Autodesk Inventor part; units mm, degrees
ref_plane "YZ Plane" through (0, 0, 0) normal (1, 0, 0) x (0, 1, 0)
ref_plane "XZ Plane" through (0, 0, 0) normal (0, 1, 0) x (-1, 0, 0)
ref_plane "XY Plane" through (0, 0, 0) normal (0, 0, 1) x (1, 0, 0)
sketch "Sketch1" plane through (0, 0, 0) normal (0, 1, 0) x (-1, 0, 0)
  line L0 (0, 0) -> (50, 0)
  line L1 (50, 0) -> (50, -155)
  line L2 (50, -155) -> (0, -155)
  line L3 (0, -155) -> (0, 0)
  dimension "d0" = 155
  dimension "d1" = 50
extrude "Extrusion1" add sketch "Sketch1" along normal blind 5
sketch "Sketch2" plane through (0, 0, 0) normal (0, -1, 0) x (1, 0, 0)
  line L0 (-6, -6.5) -> (-44, -6.5)
  line L1 (-44, -6.5) -> (-44, -148.5)
  line L2 (-44, -148.5) -> (-6, -148.5)
  line L3 (-6, -148.5) -> (-6, -6.5)
  line L4 (0, 0) -> (0, -155)
  line L5 (0, -155) -> (-50, -155)
  dimension "d4" = 38
  dimension "d5" = 142
  dimension "d6" = 6
  dimension "d7" = 6.5
extrude "Extrusion2" add sketch "Sketch2" along normal blind 5
ref_plane "Work Plane1" through (-25, 0, 0) normal (1, 0, 0) x (0, 0, -1)
sketch "Sketch3" plane through (-25, 0, 0) normal (1, 0, 0) x (0, 0, -1)
  line L0 (155, 5) -> (0, 5)
  arc A0 (97.5, 5) -> (57.5, 5) centre (77.5, 5) ccw
  arc A1 (92.5, 5) -> (62.5, 5) centre (77.5, 5) ccw
  point P0 (0, 0)
  point P1 (73.9182, 2.8954)
  point P2 (77.5, 5)
  point P3 (77.5, 5)
  point P4 (77.5, 25)
  point P5 (77.5, 20)
  dimension "d11" = 77.5
  dimension "d12" = 0
  dimension "d13" = 20
  dimension "d14" = 20
  dimension "d15" = 20
  dimension "d16" = 5
  dimension "d17" = 5
  dimension "d18" = 5
extrude "Extrusion3" add sketch "Sketch3" along normal mid plane 5 contours L0 A1 A0
chamfer "Chamfer1" distance 2 angle 45 4 edges at (-22.5, 25, -77.5) (-27.5, 25, -77.5) (-22.5, 20, -77.5) (-27.5, 20, -77.5)
chamfer "Chamfer2" distance 1 angle 45 8 edges at (0, 5, -77.5) (-25, 5, -155) (-50, 5, -77.5) (-25, 5, 0) (-25, 0, -155) (0, 0, -77.5) (-50, 0, -77.5) (-25, 0, 0)
chamfer "Chamfer3" distance 1 angle 45 4 edges at (-25, -5, -6.5) (-44, -5, -77.5) (-6, -5, -77.5) (-25, -5, -148.5)
equation "\"BendRadius\" = Thickness"
equation "\"BendReliefWidth\" = Thickness"
equation "\"BendReliefDepth\" = 0.5 * Thickness"
equation "\"CornerReliefSize\" = 4 * Thickness"
equation "\"MinimumRemnant\" = 2 * Thickness"
equation "\"TransitionRadius\" = BendRadius"
equation "\"JacobiRadiusSize\" = BendRadius"
equation "\"GapSize\" = Thickness"
properties part number "water lock"
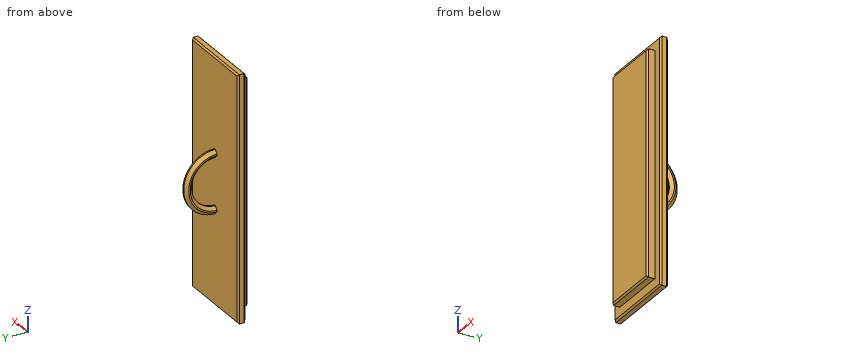
Source: CAD feature listing. Evaluate the final solid. Frame: model axes, mm. Give positions to 0.01 mm unless a question says otherwise; leave off trailing zeros. Write each loop counter-clockwise with the first axis right and the second up, starting at its lowest first coordinate (ties: lowest second). Pieces come first, ordered by that corner, then holes. Notation, with made-up numbers: (13, 46.25) - (69, 46.25) arc R32 cw to (69, 76.25) - close; hole circle Ø7 at (46, -11). An arc over 180 degrees is marked (long way). Write item = value, one per line. Start each with the question number.
Q1. Material intervals for probe 1 along Y at (x, z) = (-32, -144.5); probe 2 along X at (y, z) = (-1, -46); probe 3 along Z at (x, y) = (-24.5, 15), sorted ascending.
Q2. Pin query (flat end, axial travel): pin 1 Ø1.5 at (y, z) = (5.5, -34) entering from -X; pin 2 Ø1.5 at (y, z) = (-1, -127.5) entering from +X; pin 3 Ø14.5 at (y, z) = (13, -76) entering from -X. Return the tip coordinate at first contact, or that it passes through.
Q3. Cut plane A-A, the plane z = -77.5. Return loops of the section in (x, y).
Q4. Cut plane B-B, the plane z = -39. Return loops of the section in (x, y), then the cut area to 3 significant figures.
Computed values:
q1.probe_1 = -5 to 5
q1.probe_2 = -44 to -6
q1.probe_3 = -94.82 to -88.68, -66.32 to -60.18
q2.pin_1 = -49.25
q2.pin_2 = -6
q2.pin_3 = -25.89
q3.outline = (-50, 1) - (-49, 0) - (-44, 0) - (-44, -4) - (-43, -5) - (-7, -5) - (-6, -4) - (-6, 0) - (-1, 0) - (0, 1) - (0, 4) - (-1, 5) - (-49, 5) - (-50, 4) - close; (-27.5, 22) - (-25.5, 20) - (-24.5, 20) - (-22.5, 22) - (-22.5, 23) - (-24.5, 25) - (-25.5, 25) - (-27.5, 23) - close
q4.outline = (-50, 1) - (-49, 0) - (-44, 0) - (-44, -4) - (-43, -5) - (-7, -5) - (-6, -4) - (-6, 0) - (-1, 0) - (0, 1) - (0, 4) - (-1, 5) - (-49, 5) - (-50, 4) - close
q4.area = 437 mm²
